```python
from build123d import *

# Parameters (mm, degrees)
SKETCH_1_R                = 4.5
EXTRUDE_1_DEPTH           = 13
CUT_EXTRUDE_1_DEPTH       = 6.5
CUT_EXTRUDE_2_DEPTH       = 6.5
SKETCH_4_R                = 1
CUT_EXTRUDE_3_DEPTH       = 6.5
HOLE_WIZARD_1_D           = 3
HOLE_WIZARD_1_CSINK_D     = 3.5
HOLE_WIZARD_1_CSINK_ANGLE = 90
CHAMFER_1_SIZE            = 0.5
HOLE_WIZARD_M3_1_REACH    = 18.439
HOLE_WIZARD_M3_1_BORE_R   = 1.25


with BuildPart() as part:
    # 草图1 → 凸台-拉伸1 (new body)
    with BuildSketch(Plane.XY):
        with Locations(Location((0, 0, 0), (0, 0, 180))):
            Circle(SKETCH_1_R)
    extrude(amount=EXTRUDE_1_DEPTH)

    # 草图2 → 切除-拉伸1 (cut, symmetric)
    with BuildSketch(Plane(origin=(0, 0, 0), x_dir=(1, 0, 0), z_dir=(0, 1, 0))):
        with BuildLine():
            Line((5e-09, 0), (-4.5, 0))
            Line((-4.5, 0), (-4.5, -9))
            ThreePointArc((-4.5, -9), (-2.732233047, -8.267766953), (-2, -6.5))
            Line((-2, -6.5), (-2, -2))
            ThreePointArc((-2, -2), (-1.414213561, -0.585786436), (5e-09, 0))
        make_face()
        with BuildLine():
            Line((4.5, 0), (5e-09, 0))
            ThreePointArc((5e-09, 0), (1.414213564, -0.585786439), (2, -2))
            Line((2, -2), (2, -6.5))
            ThreePointArc((2, -6.5), (2.732233047, -8.267766953), (4.5, -9))
            Line((4.5, -9), (4.5, 0))
        make_face()
    extrude(amount=CUT_EXTRUDE_1_DEPTH, both=True, mode=Mode.SUBTRACT)

    # 草图3 → 切除-拉伸2 (cut, symmetric)
    with BuildSketch(Plane(origin=(0, 0, 0), x_dir=(0, 0, -1), z_dir=(1, 0, 0))):
        with BuildLine():
            Line((0, 3), (-5, 3))
            ThreePointArc((-5, 3), (-7.16227766, 0), (-5, -3))
            Line((-5, -3), (0, -3))
            Line((0, -3), (0, 3))
        make_face()
    extrude(amount=CUT_EXTRUDE_2_DEPTH, both=True, mode=Mode.SUBTRACT)

    # 草图4 → 切除-拉伸3 (cut, symmetric)
    with BuildSketch(Plane(origin=(0, 0, 0), x_dir=(1, 0, 0), z_dir=(0, 1, 0))):
        with Locations(Location((0, -1.778928225, 0), (0, 0, 270))):
            Circle(SKETCH_4_R)
    extrude(amount=CUT_EXTRUDE_3_DEPTH, both=True, mode=Mode.SUBTRACT)

    # 打孔尺寸根据开槽半沉头木螺钉的类型1 (through all)
    with Locations(Plane.XY.offset(13)):
        with Locations((0, 0)):
            CounterSinkHole(HOLE_WIZARD_1_D / 2, HOLE_WIZARD_1_CSINK_D / 2, counter_sink_angle=HOLE_WIZARD_1_CSINK_ANGLE)

    # 倒角1
    chamfer_1_edges = [part.edges().sort_by_distance(p)[0] for p in [
        (4.5, 0, 13),
    ]]
    chamfer(chamfer_1_edges, length=CHAMFER_1_SIZE)

    # M3 螺纹孔1 bore → M3 螺纹孔1 (cut, up to next)
    with BuildSketch(Plane(origin=(0, 4.5, 0), x_dir=(1, 0, 0), z_dir=(0, 1, 0)), mode=Mode.PRIVATE) as hole_wizard_m3_1_sk1:
        with Locations((0, -10.5)):
            Circle(HOLE_WIZARD_M3_1_BORE_R)
    hole_wizard_m3_1_tool1 = extrude(hole_wizard_m3_1_sk1.sketch, amount=-HOLE_WIZARD_M3_1_REACH, mode=Mode.PRIVATE) & part.part
    add(hole_wizard_m3_1_tool1.solids().sort_by_distance((0, 4.5, 10.5))[0], mode=Mode.SUBTRACT)


solid = part.part
```
Geometry check sheet. Reference: the model listing, model coordinates, mm. A direction names the side the tool comes from. Coordinates: 2 decimals unless noted, no trailing zeros. Order: outer loops, then holes, each group sorted by start corner. A loop starts at its lowest first (then second) coordinate and runs counter-clockwise, first axis right, second up. Notation, with made-up numbers: (-30.5, 25) - (5.5, 25) arc R11 ccw to (5.5, 35) - close; hole circle Ø7 at (-30.75, 36). An arc over 180 degrees is marked (long way). Answer as a JSON object with one key per item and string values. Group by question number.
Item 1: Draft check along X on faces 1 (the face through (3.32, -3.04, 8.94)), 2 (the face through (0.325, -1.464, 9.725)), 3 (the face through (0, 3, 3)). Enter one of: +X half, -X half, draft (parallel to the pull), parting line (faces both ways), or undercut.
Item 2: Sectioned sample at B-B, the plane y = 0. Record the cut outline in (x, z), and give its area (3 significant figures).
Item 3: Sectioned sample at D-D, the plane x = 0.25. Give the number of separate pieces and of enclosed holes in the cut face, and give its area (3 significant figures).
Item 4: Tool access check on faces 4 (the face through (-2, -3.4, 4.8)), 5 (the face through (1.19, 2.69, 10.12)), 6 (the face through (0, -3, 3)), 7 (the face through (2, -3.4, 4.7)). Record the directions out of +Z, -Z, +X, -X, +Y, -Y that give a thin tool (end or side, any length) a straight path to the whole face; none if there is none.
Item 5: Depth check by flat-ended pin: pin 1 Ø1 at (y, z) = (1.5, 9) entering from +X; pin 2 Ø0.6 at (y, z) = (-3, 4.5) entering from -X; pin 3 Ø1 at (x, y) = (-3, 0) entering from -Z. Enter the tip coordinate at first touch or a pass-through.
Item 6: Sectioned sample at A-A, the plane z = 4.75. Record the cut outline in (x, y), and give its area (3 significant figures).
Item 7: Sectioned sample at C-C, the plane z = 2.5. Record the cut outline in (x, y).
Item 8: Scan lines: probe 1 along Y at (x, z) = (0, 10); probe 2 along X at (y, z) = (0.75, 8.5); probe 3 along Z at (x, y) = (-1, 2). Record each from-to range of solid material in increasing order.
Resolved:
{
 "1": {"face 1": "parting line", "face 2": "undercut", "face 3": "draft"},
 "2": {"outline": "(-4.5, 9) arc R2.5 cw to (-2.09, 7.16) - (-1.5, 7.16) - (-1.5, 12.75) - (-1.75, 13) - (-4, 13) - (-4.5, 12.5) - close; (1.5, 7.16) - (2.09, 7.16) arc R2.5 cw to (4.5, 9) - (4.5, 12.5) - (4, 13) - (1.75, 13) - (1.5, 12.75) - close", "area": "28.2 mm^2"},
 "3": {"separate pieces": "5", "enclosed holes": "0", "area": "46.2 mm^2"},
 "4": {"face 4": "-Z, -X, +Y, -Y", "face 5": "+Y", "face 6": "-Z, +X, -X", "face 7": "-Z, +X, +Y, -Y"},
 "5": {"pin 1": "x = 4.39", "pin 2": "x = -2", "pin 3": "z = 8"},
 "6": {"outline": "(-2, -4.03) arc R4.5 ccw to (2, -4.03) - (2, -3) - (-2, -3) - close; (-2, 3) - (2, 3) - (2, 4.03) arc R4.5 ccw to (-2, 4.03) - close", "area": "10.8 mm^2"},
 "7": {"outline": "(-2, -4.03) arc R4.5 ccw to (-0.69, -4.45) - (-0.69, -3) - (-2, -3) - close; (-2, 3) - (-0.69, 3) - (-0.69, 4.45) arc R4.5 ccw to (-2, 4.03) - close; (0.69, -4.45) arc R4.5 ccw to (2, -4.03) - (2, -3) - (0.69, -3) - close; (0.69, 3) - (2, 3) - (2, 4.03) arc R4.5 ccw to (0.69, 4.45) - close"},
 "8": {"probe 1": "-4.5 to -1.5", "probe 2": "-3 to -1.3, 1.3 to 3", "probe 3": "6.45 to 9.75, 11.25 to 13"}
}
